The listing builds one solid part. Answer for the finished solid, in the listing's coordinates (mm). Face numbers are marked on the shaded views. A direction names the side the tool comes from. Coordinates: 2 decimals unless noted, no trailing zeros. Order: outer loops, then holes, each group sorted by start corner. A loop starts at its lowest first (then second) coordinate and runs counter-clockwise, first axis right, second up.
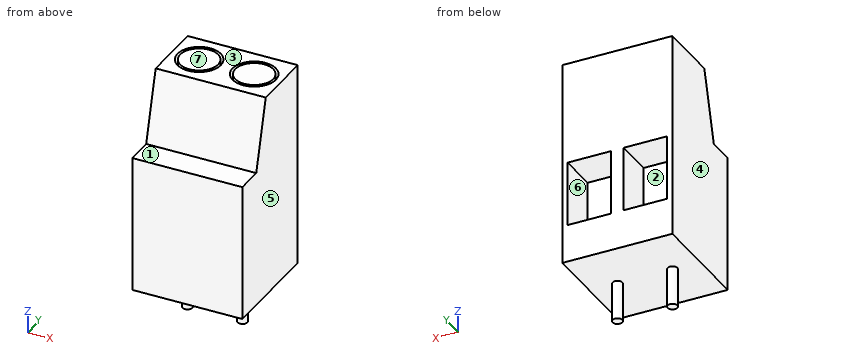
Autodesk Inventor part; units mm, degrees
ref_plane "YZ Plane" through (0, 0, 0) normal (1, 0, 0) x (0, 1, 0)
ref_plane "XZ Plane" through (0, 0, 0) normal (0, 1, 0) x (-1, 0, 0)
ref_plane "XY Plane" through (0, 0, 0) normal (0, 0, 1) x (1, 0, 0)
sketch "Sketch1" plane through (0, 0, 0) normal (1, 0, 0) x (0, 1, 0)
  line L0 (-6.9022, 3.3081) -> (3.0978, 3.3081)
  line L1 (3.0978, 3.3081) -> (3.0978, -9.3586)
  line L2 (3.0978, -9.3586) -> (-6.9022, -9.3586)
  line L3 (-6.9022, -9.3586) -> (-6.9022, 3.3081)
  line L4 (-4.3921, 3.3081) -> (-2.6747, 9.6414)
  line L5 (-2.6747, 9.6414) -> (3.0978, 9.6414)
  line L6 (3.0978, 9.6414) -> (3.0978, 3.3081)
  point P0 (0, 0)
  dimension "d0" = 10
  dimension "d1" = 19
  dimension "d2" = 12.6667
extrude "Extrusion1" add sketch "Sketch1" along normal blind 10.16
sketch "Sketch2" plane through (0, -6.9022, -9.3586) normal (0, 0, -1) x (-1, 0, 0)
  line L0 (-10.16, 0) -> (-10.16, 10)
  line L1 (0, 0) -> (-10.16, 0)
  circle A0 centre (-7.62, 5) radius 0.45
  circle A1 centre (-2.54, 5) radius 0.45
  point P0 (0, 6.9022)
  dimension "d5" = 0.9
  dimension "d6" = 0.9
  dimension "d7" = 5.08
  dimension "d8" = 2.54
  dimension "d9" = 5
  dimension "d10" = 5
extrude "Extrusion2" add sketch "Sketch2" along normal blind 3.6
sketch "Sketch3" plane through (0, -2.6747, 9.6414) normal (0, 0, 1) x (1, 0, 0)
  line L0 (0, 5.7725) -> (0, 0)
  circle A0 centre (2.54, 2.8863) radius 2
  circle A1 centre (7.62, 2.8863) radius 2
  point P0 (0, 2.6747)
  dimension "d13" = 5.08
  dimension "d14" = 4
  dimension "d15" = 4
  dimension "d16" = 2.54
extrude "Extrusion3" cut sketch "Sketch3" against normal blind 3.6
sketch "Sketch4" plane through (2.54, 0.2116, 6.0414) normal (0, 0, 1) x (1, 0, 0)
  circle A0 centre (0, 0) radius 2
  circle A1 centre (0, 0) radius 1.75
  circle A2 centre (5.08, 0) radius 1.75
  point P0 (-2.54, -0.2116)
  dimension "d19" = 5.08
  dimension "d20" = 3.5
  dimension "d21" = 3.5
extrude "Extrusion4" add sketch "Sketch4" along normal blind 3.6 contours A1 | A2
sketch "Sketch5" plane through (0, 3.0978, 9.6414) normal (0, 1, 0) x (1, 0, 0)
  line L0 (0, 19) -> (0, 0)
  line L1 (10.16, 19) -> (10.16, 0)
  line L2 (0, 19) -> (10.16, 19)
  line L3 (0.5, 15.5) -> (4.5, 15.5)
  line L4 (4.5, 15.5) -> (4.5, 9.5)
  line L5 (4.5, 9.5) -> (0.5, 9.5)
  line L6 (0.5, 9.5) -> (0.5, 15.5)
  line L7 (5.66, 15.5) -> (9.66, 15.5)
  line L8 (9.66, 15.5) -> (9.66, 9.5)
  line L9 (9.66, 9.5) -> (5.66, 9.5)
  line L10 (5.66, 9.5) -> (5.66, 15.5)
  point P0 (0, 9.6414)
  dimension "d24" = 4
  dimension "d25" = 4
  dimension "d26" = 0.5
  dimension "d27" = 0.5
  dimension "d28" = 3.5
  dimension "d29" = 3.5
  dimension "d30" = 6
  dimension "d31" = 6
extrude "Extrusion5" cut sketch "Sketch5" against normal blind 3.6
properties part number "ScrewTerminal"
(1) Given pin 1 Ø2.5 at (x, y) = (7.62, 0.21) entering from -Z; pin 2 Ø1.5 at (x, z) = (4.5, 6.5) entering from -Y, each flat-ended and moving along its own axis, determine where each tip first touches the part or whether it passes through.
(2) Find section A-A on x = 7.62. Determine the outline of the cut face in (y, z).
(3) Find section D-D on z = 5. Determine the outline of the cut face in (x, y), then the cut area to 3 significant figures.
(4) A tool of negligible diameter and unlimited length cuts with its end or side. For the marked faces 1, 2 and 3, from which of +Z, -Z, +X, -X, +Y, -Y can it reach the whole face along a straight path? Write none if from no direction.
(5) Find the intervals of material crossed by probe 1 along X at (y, z) = (1, -3); probe 2 along Y at (x, z) = (2.54, 7.2); probe 3 along Y at (x, z) = (7.62, 7.55), in increasing order.
(6) Find section B-B on z = -1. Determine the outline of the cut face in (x, y).
(7) The mould has two halves that part along X. Classify the marked faces 4, 5, 6 and 7: pulls with the +X half, pulls with the -X half, needs draft (parallel to the pull), parting line crosses it, or undercut.
(8) Find section C-C on y = -0.25. Determine the outline of the cut face in (x, z), then the cut area to 3 significant figures.
Resolved:
1. pin 1: stops at z = -9.36
1. pin 2: stops at y = -3.73
2. outline: (-6.9, -9.36) - (-2.35, -9.36) - (-2.35, -12.96) - (-1.45, -12.96) - (-1.45, -9.36) - (3.1, -9.36) - (3.1, -5.86) - (-0.5, -5.86) - (-0.5, 0.14) - (3.1, 0.14) - (3.1, 9.64) - (2.21, 9.64) - (2.21, 6.04) - (1.96, 6.04) - (1.96, 9.64) - (-1.54, 9.64) - (-1.54, 6.04) - (-1.79, 6.04) - (-1.79, 9.64) - (-2.67, 9.64) - (-4.39, 3.31) - (-6.9, 3.31) - close
3. outline: (0, -3.93) - (10.16, -3.93) - (10.16, 3.1) - (0, 3.1) - close
3. area: 71.4 mm2
4. face 1: +Z, +X, -X, -Y
4. face 2: +Y
4. face 3: +Z, +X, -X, +Y, -Y
5. probe 1: x = 0 to 0.5, 4.5 to 5.66, 9.66 to 10.16
5. probe 2: y = -3.34 to -1.79, -1.54 to 1.96, 2.21 to 3.1
5. probe 3: y = -3.24 to -1.79, -1.54 to 1.96, 2.21 to 3.1
6. outline: (0, -6.9) - (10.16, -6.9) - (10.16, 3.1) - (9.66, 3.1) - (9.66, -0.5) - (5.66, -0.5) - (5.66, 3.1) - (4.5, 3.1) - (4.5, -0.5) - (0.5, -0.5) - (0.5, 3.1) - (0, 3.1) - close
7. face 4: pulls with the -X half
7. face 5: pulls with the +X half
7. face 6: undercut
7. face 7: needs draft
8. outline: (0, -9.36) - (10.16, -9.36) - (10.16, 9.64) - (9.57, 9.64) - (9.57, 6.04) - (9.31, 6.04) - (9.31, 9.64) - (5.93, 9.64) - (5.93, 6.04) - (5.67, 6.04) - (5.67, 9.64) - (4.49, 9.64) - (4.49, 6.04) - (4.23, 6.04) - (4.23, 9.64) - (0.85, 9.64) - (0.85, 6.04) - (0.59, 6.04) - (0.59, 9.64) - (0, 9.64) - close; hole (0.5, -5.86) - (4.5, -5.86) - (4.5, 0.14) - (0.5, 0.14) - close; hole (5.66, -5.86) - (9.66, -5.86) - (9.66, 0.14) - (5.66, 0.14) - close
8. area: 141 mm2
